Autodesk Inventor part; units mm, degrees
ref_plane "YZ Plane" through (0, 0, 0) normal (1, 0, 0) x (0, 1, 0)
ref_plane "XZ Plane" through (0, 0, 0) normal (0, 1, 0) x (-1, 0, 0)
ref_plane "XY Plane" through (0, 0, 0) normal (0, 0, 1) x (1, 0, 0)
sketch "Sketch1" plane through (0, 0, 0) normal (0, 1, 0) x (-1, 0, 0)
  line L0 (0, 0) -> (133.35, 0)
  line L1 (133.35, 0) -> (133.35, -133.35)
  line L2 (133.35, -133.35) -> (0, -133.35)
  line L3 (0, -133.35) -> (0, 0)
  line L4 (66.675, 0) -> (66.675, -66.675)
  line L5 (1.905, -1.905) -> (131.445, -1.905)
  line L6 (131.445, -1.905) -> (131.445, -131.445)
  line L7 (131.445, -131.445) -> (1.905, -131.445)
  line L8 (1.905, -131.445) -> (1.905, -1.905)
  line L9 (1.905, -1.905) -> (131.445, -131.445) construction
  line L10 (131.445, -1.905) -> (1.905, -131.445) construction
  dimension "d0" = 133.35
  dimension "d1" = 133.35
  dimension "d2" = 66.675
  dimension "d3" = 129.54
  dimension "d4" = 129.54
extrude "Extrusion1" add sketch "Sketch1" along normal blind 2.54 contours L5 L6 L7 L8
extrude "Extrusion2" add sketch "Sketch1" against normal blind 2.54 contours L5 L6 L7 L8 | L0 L1 L2 L3
fillet "Fillet1" radius 1.27 4 edges at (-133.35, -2.54, -66.675) (-66.675, -2.54, -133.35) (-66.675, -2.54, 0) (0, -2.54, -66.675)
properties part number "TC720 lid"
Could you check a few things on this model? Use its own coordinates, in mm. Coordinates: 2 decimals unless noted, no trailing zeros. Write each loop counter-clockwise with the first axis right and the second up, starting at its lowest first coordinate (ties: lowest second). Pieces come first, ordered by that corner, then holes. Notation, with made-up numbers: (82.25, 22) -> (89.25, 22) arc R21 ccw to (89.25, 31) -> close; hole circle Ø9 at (-37, -23.5). An arc over 180 degrees is marked (long way). Write item = value, one per line. Start each with the question number.
(1) I want a section at C-C (y = 1). Please give me the cut outline in (x, z) (3 decimals), plus the area to 3 significant figures.
(2) Will these pins go through, and if not, where does the flat tip stop? pin 1 (2 mm diameter, centred on x = -75, y = 1.5, fed in from +Z) (3 decimals); pin 2 (0.8 mm diameter, centred on x = -46.5, y = 1, fed in from -Z) (3 decimals); pin 3 (3 mm diameter, centred on y = 2, z = -85.5, fed in from +X) (3 decimals).
(3) I want a section at B-B (x = -101). Please give me the cut outline in (y, z) (3 decimals).
(4) I want a section at A-A (z = -26). Please give me the cut outline in (x, y) (3 decimals).
(5) I need wall thicknesses on line 1 (Z direction, x = -60, y = 0.6) (3 decimals); line 2 (Z direction, x = -43, y = -1.35). Which ranges of each line are inside material? Lowest first, please. Write a range as [from, to].
Result set:
q1.outline = (-131.445, -131.445) -> (-1.905, -131.445) -> (-1.905, -1.905) -> (-131.445, -1.905) -> close
q1.area = 16,800 mm2
q2.pin_1 = -1.905
q2.pin_2 = -131.445
q2.pin_3 = -1.905
q3.outline = (-2.54, -132.08) arc R1.27 ccw to (-1.27, -133.35) -> (0, -133.35) -> (0, -131.445) -> (2.54, -131.445) -> (2.54, -1.905) -> (0, -1.905) -> (0, 0) -> (-1.27, 0) arc R1.27 ccw to (-2.54, -1.27) -> close
q4.outline = (-133.35, -1.27) arc R1.27 ccw to (-132.08, -2.54) -> (-1.27, -2.54) arc R1.27 ccw to (0, -1.27) -> (0, 0) -> (-1.905, 0) -> (-1.905, 2.54) -> (-131.445, 2.54) -> (-131.445, 0) -> (-133.35, 0) -> close
q5.line_1 = [-131.445, -1.905]
q5.line_2 = [-133.35, 0]
